Answer from the drawing. Dimensions are ordinates in mm from the lowest x, y and z of the part. Give positions to 0.01 mm unless a question says otherwise; leave off trailing zeros. Order: outer loops, then holes, each group sorted by start corner. A loop starts at its lowest first (then second) coordinate and runs counter-clockwise, first axis right, second up. Notation, with made-up numbers: (67.5, -3.5) - (109.5, -3.5) arc R32 ccw to (109.5, 28.5) - close; hole circle Ø4 at (-35, -15.5). An arc over 180 degrees is marked (long way). Answer in a Markdown table with one row per item.
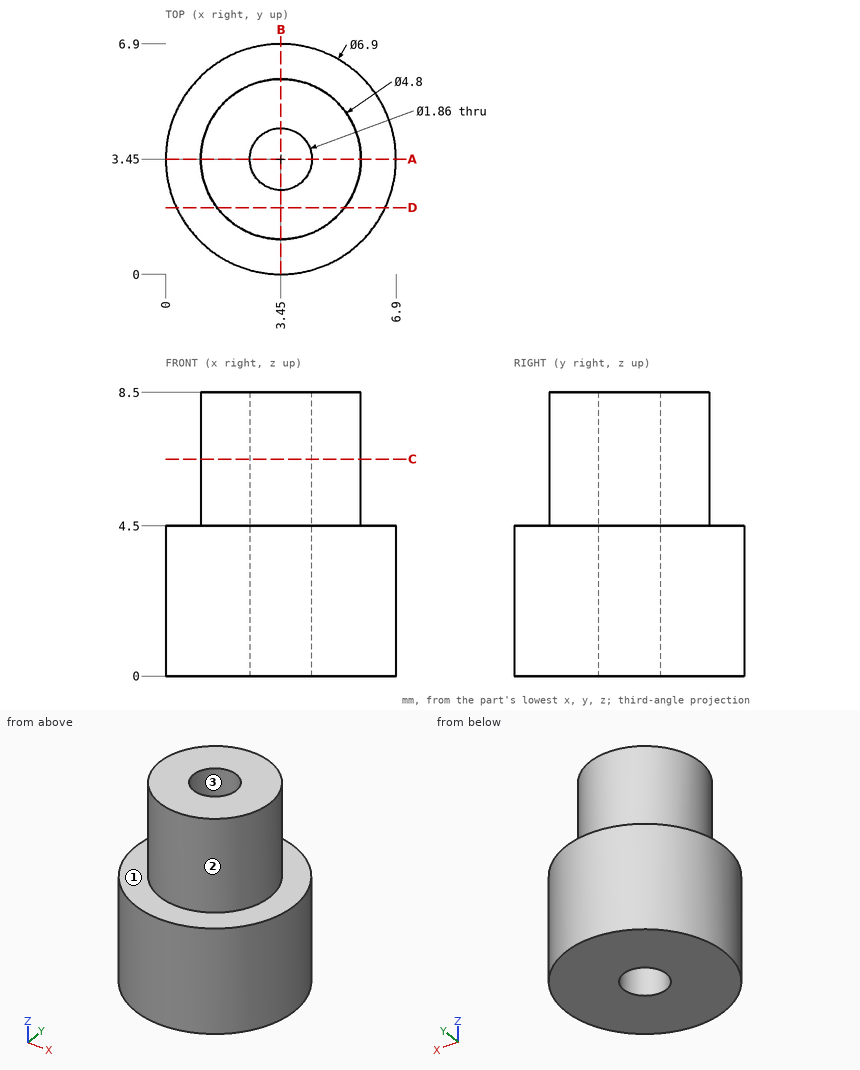
Item 1: Find section D-D on y = 2. Write down the section's boundary in (x, z).
Answer block:
| item | result |
|---|---|
| outline | (0.32, 0) - (6.58, 0) - (6.58, 4.5) - (5.36, 4.5) - (5.36, 8.5) - (1.54, 8.5) - (1.54, 4.5) - (0.32, 4.5) - close |
Item 2: Find section C-C on z = 6.5. Write down the section's boundary in (x, y).
Answer block:
| item | result |
|---|---|
| outline | circle Ø4.8 at (3.45, 3.45); hole circle Ø1.86 at (3.45, 3.45) |
Item 3: Find section A-A on y = 3.45. Write down the section's boundary in (x, z), then the cut area to 3 significant figures.
Answer block:
| item | result |
|---|---|
| outline | (0, 0) - (2.52, 0) - (2.52, 8.5) - (1.05, 8.5) - (1.05, 4.5) - (0, 4.5) - close; (4.38, 0) - (6.9, 0) - (6.9, 4.5) - (5.85, 4.5) - (5.85, 8.5) - (4.38, 8.5) - close |
| area | 34.4 mm² |
Item 4: Each of these flat-tipped pins is pushed along its axis until it touches: P1, Ø3, axis at y = 5, z = 4, coming from the -X side; P2, Ø1, axis at x = 4, z = 6, coming from the +Y side; P3, Ø2, axis at x = 1, z = 6, coming from the -Y side; P4, Ø1.7, axis at x = 3.45, y = 3.45, coming from the +Z side. Where does it stop, or does it pass through?
Answer block:
| item | result |
|---|---|
| P1 | x = 0 |
| P2 | y = 5.85 |
| P3 | y = 1.54 |
| P4 | through |
Item 5: Consider line 1 (Y direction, x = 3.45, z = 6.75); line 2 (Y direction, x = 3.5, z = 3.25). Determine where each line is inside the solid, lowest interval first.
Answer block:
| item | result |
|---|---|
| line 1 | 1.05 to 2.52, 4.38 to 5.85 |
| line 2 | 0 to 2.52, 4.38 to 6.9 |
Item 6: Determine the mould class of the marked faces 1, 2 and 3 for opening direction Y: pulls with the +Y half, pulls with the -Y half, needs draft (parallel to the pull), parting line crosses it, or undercut.
Answer block:
| item | result |
|---|---|
| face 1 | needs draft |
| face 2 | parting line crosses it |
| face 3 | undercut |
